```python
from build123d import *

# Parameters (mm, degrees)
BOSS_EXTRUDE1_DEPTH      = 12.7
BOSS_EXTRUDE1_DEPTH_BACK = 12.7
CUT_EXTRUDE1_DEPTH       = 35.478524438


with BuildPart() as part:
    # Sketch1 → Boss-Extrude1 (new, two sides: drawn at the far end of the back side and taken through both)
    with BuildSketch(Plane(origin=(0, 0, 0), x_dir=(1, 0, 0), z_dir=(0, 1, 0)).offset(-BOSS_EXTRUDE1_DEPTH_BACK)):
        Polygon((-24.645544554, -5.847029703), (0.754455446, -5.847029703), (0.754455446, 19.552970297), (-5.595544554, 19.552970297), (-5.595544554, 0.502970297), (-18.295544554, 0.502970297), (-18.295544554, 19.552970297), (-24.645544554, 19.552970297), align=None)
    extrude(amount=BOSS_EXTRUDE1_DEPTH + BOSS_EXTRUDE1_DEPTH_BACK)

    # Sketch3 → Cut-Extrude1 (cut, through all)
    with BuildSketch(Plane.ZY.offset(24.645544554)):
        with BuildLine():
            ThreePointArc((-10.027970297, 3.175), (-13.202970297, 0), (-10.027970297, -3.175))
            Line((-10.027970297, -3.175), (-10.027970297, 0))
            Line((-10.027970297, 0), (-10.027970297, 3.175))
        make_face()
        with BuildLine():
            Line((-10.027970297, 0), (-10.027970297, -3.175))
            ThreePointArc((-10.027970297, -3.175), (-7.782906267, -2.24506403), (-6.852970297, 0))
            ThreePointArc((-6.852970297, 0), (-7.782906267, 2.24506403), (-10.027970297, 3.175))
            Line((-10.027970297, 3.175), (-10.027970297, 0))
        make_face()
    extrude(amount=-CUT_EXTRUDE1_DEPTH, mode=Mode.SUBTRACT)


solid = part.part
```
Here's how the part is built. I have some questions about the finished solid (model axes, mm). A direction names the side the tool comes from. Give positions to 0.01 mm unless a question says otherwise; leave off trailing zeros. Loops run counter-clockwise (first coordinate to the right, second up) from the corner with the lowest first, then second, coordinate; pieces in that order, holes last. Notation, with made-up numbers: M 56.5,72.5 L 115.5,72.5 A27 cw 115.5,94.5 Z; hole C -17,85.25 d6. An arc over 180 degrees is marked long. Put each result on its own line as item: value. Start each with the question number.
(1) I want a section at A-A on z = -14.25. Please give me the cut outline in (x, y).
(2) I want a section at B-B on x = -1.25. Please give me the cut outline in (y, z) (3 decimals).
(3) Will this pin go through, and if not, where does the flat tip stop? pin 1 Ø12 at (x, y) = (-17.5, 9) entering from -Z.
(4) I want a section at D-D on x = -11.5. Please give me the cut outline in (y, z), then the cut area to 3 significant figures.
(5) I want a section at C-C on y = -5.25. Please give me the cut outline in (x, z).
(6) For faces 4 (the flat face through (-5.596, -3, -8)), 5 (the flat face through (-21, 0, -19.553)), which set-ups out of +Z, -Z, +X, -X, +Y, -Y let a thin tool reach every point of the face, with its end or its side?
(7) I need wall thicknesses on line 1 along X through (y, z) = (-6, -8.5); line 2 along Y through (x, z) = (-1.5, -8); line 3 along Y through (x, z) = (-4, -9). Which ranges of each line are inside material? Lowest first, please. Write a range as [from, to].
(8) If we mould it in two halves opening along X, with no side actions, what happens to faces 1 (the flat face through (0.754, -0.2, -6.7)), 2 (the flat face through (-18.296, 3, -8)), 3 (the flat face through (-2, 0, -19.553))? For each: +X half, -X half, draft (parallel to the pull), parting line (faces both ways), or undercut.
Answer block:
1. outline: M -24.65,-12.7 L -18.3,-12.7 L -18.3,12.7 L -24.65,12.7 Z; M -5.6,-12.7 L 0.75,-12.7 L 0.75,12.7 L -5.6,12.7 Z
2. outline: M -12.7,-19.553 L 12.7,-19.553 L 12.7,5.847 L -12.7,5.847 Z; hole C 0,-10.028 d6.35
3. pin 1: z = -19.55
4. outline: M -12.7,-0.5 L 12.7,-0.5 L 12.7,5.85 L -12.7,5.85 Z
4. area: 161 mm^2
5. outline: M -24.65,-19.55 L -18.3,-19.55 L -18.3,-0.5 L -5.6,-0.5 L -5.6,-19.55 L 0.75,-19.55 L 0.75,5.85 L -24.65,5.85 Z
6. face 4: -Z, +Y, -Y
6. face 5: -Z, +X, -X, +Y, -Y
7. line 1: [-24.65, -18.3], [-5.6, 0.75]
7. line 2: [-12.7, -2.44], [2.44, 12.7]
7. line 3: [-12.7, -3], [3, 12.7]
8. face 1: +X half
8. face 2: undercut
8. face 3: draft
